Geometry check sheet. Reference: the model listing, model coordinates, mm. Give positions to 0.01 mm unless a question says otherwise; leave off trailing zeros. Order: outer loops, then holes, each group sorted by start corner. A loop starts at its lowest first (then second) coordinate and runs counter-clockwise, first axis right, second up. Notation, with made-up numbers: M 12.25,37 L 52.25,37 A11 cw 52.25,42 Z; hole C 61.25,55.5 d6. An arc over 180 degrees is marked long. Answer as CSV lines item,"result". Start each with the question number.
Q1. Thickness scan on line 1 (Y direction, x = -7, z = 2.25); line 2 (Z direction, x = 70, y = -56.5); line 3 (Y direction, x = 75, z = -2). Record the ranges inside material, lowest first.
Q2. Section check A-A, the plane x = 0. Record the boundary of the cut face in (y, z).
Q3. Go/stop test with flat-tipped pins: pin 1 (6 mm diameter, centred on x = 58.5, z = 2.5, fed in from +Y); pin 2 (1 mm diameter, centred on y = -27.5, z = 3.5, fed in from -X); pin 3 (1.5 mm diameter, centred on x = 23.5, z = 0, fed in from -Y). Record where each tip stops, or that it passes through.
Q4. Section check B-B, the plane z = 6.5. Record the boundary of the cut face in (x, y), then the cut area to 3 significant figures.
Autodesk Inventor part; units mm, degrees
ref_plane "YZ Plane" through (0, 0, 0) normal (1, 0, 0) x (0, 1, 0)
ref_plane "XZ Plane" through (0, 0, 0) normal (0, 1, 0) x (-1, 0, 0)
ref_plane "XY Plane" through (0, 0, 0) normal (0, 0, 1) x (1, 0, 0)
sketch "Sketch1" plane through (0, 0, 0) normal (0, 1, 0) x (-1, 0, 0)
  circle A0 centre (0, 0) radius 15
  dimension "d0" = 30
extrude "Extrusion1" add sketch "Sketch1" along normal blind 7
sketch "Sketch2" plane through (0, 0, 0) normal (0, 0, 1) x (1, 0, 0)
  line L0 (0, -0.6683) -> (0, -150.6683)
  line L1 (0, -150.6683) -> (100, -150.6683)
  line L2 (15, 0) -> (-15, 0)
  line L3 (15, 0) -> (61.733, -24.0013) construction
  line L4 (61.733, -24.0013) -> (100, -85.3679) construction
  line L5 (100, -85.3679) -> (100, -133.998) construction
  spline S0 degree 3 poles (15, 0) (61.733, -24.0013) (100, -85.3679) (100, -133.998) knots 1 1 1 1 2 2 2 2
  line L6 (8.9554, -0.4801) -> (55.6884, -24.4814) construction
  line L7 (55.6884, -24.4814) -> (93.9554, -85.848) construction
  line L8 (93.9554, -85.848) -> (93.9554, -134.4781) construction
  spline S1 degree 3 poles (8.9554, -0.4801) (55.6884, -24.4814) (93.9554, -85.848) (93.9554, -134.4781) knots 1 1 1 1 2 2 2 2
  line L9 (100, -133.998) -> (93.9542, -133.998)
  line L10 (15, 0) -> (8.9554, 0)
  line L11 (8.9554, -0.4801) -> (8.9554, 0)
  point P0 (0, 0)
  dimension "d3" = 150
  dimension "d4" = 100
extrude "Extrusion2" add sketch "Sketch2" along normal mid plane 8
properties part number "preBuiltArm"
Answer block:
1,line 1,"y = 0 to 7"
1,line 2,"z = -4 to 4"
1,line 3,"y = -68.48 to -57.72"
2,outline,"M 0,-15 L 7,-15 L 7,15 L 0,15 Z"
3,pin 1,"stops at y = -32"
3,pin 2,"stops at x = 44.27"
3,pin 3,"stops at y = -9.85"
4,outline,"M -13.52,0 L 13.52,0 L 13.52,7 L -13.52,7 Z"
4,area,"189 mm2"
